from build123d import *

# Parameters (mm, degrees)
SKETCH1_W               = 50
SKETCH1_H               = 50
BODY_DEPTH              = 10
SKETCH2_R               = 11.5
CUT_VIEW_DEPTH          = 7
FILLETBODY_R            = 3
SKETCH3_R               = 3.75
BOLT_EXTRUDE_DEPTH      = 1
SKETCH4_R               = 1.5
BOLT_DEPTH              = 10
BOLT_DEPTH_BACK         = 16
HEX_2_DEPTH             = 2
SKETCH19_R              = 1.5
HEX_BOLT_DEPTH          = 3
SKETCH6_R               = 4
FIELD1_DEPTH            = 7
FIELD2_R                = 4
SKETCH7_R               = 2.575
PORTS1_DEPTH            = 12
SKETCH10_R              = 1.575
PORTS2_DEPTH            = 12
PORTS2_DEPTH_BACK       = 32
SKETCH11_R              = 20
SKETCH11_R_2            = 15
SEAL1_DEPTH             = 0.5
FLOWFIELD_DEPTH         = 1.5
FLOWFIELD_CHANNEL_DEPTH = 1.5
BODY_MOVE_COPY1_ANGLE   = 90
BODY_MOVE_COPY2_ANGLE   = 180
SKETCH20_R              = 2.575
CUT_EXTRUDE1_DEPTH      = 17
FILLET1_R               = 0.5


with BuildPart() as part:
    # Sketch1 → Body (new body)
    with BuildSketch(Plane(origin=(0, 0, 0), x_dir=(1, 0, 0), z_dir=(0, 1, 0))):
        Rectangle(SKETCH1_W, SKETCH1_H)
    extrude(amount=BODY_DEPTH)

    # Sketch2 → Cut view (cut)
    with BuildSketch(Plane(origin=(0, 10, 0), x_dir=(1, 0, 0), z_dir=(0, 1, 0))):
        Circle(SKETCH2_R)
    extrude(amount=-CUT_VIEW_DEPTH, mode=Mode.SUBTRACT)

    # FilletBody
    filletbody_edges = [part.edges().sort_by_distance(p)[0] for p in [
        (-25, 5, -25),
        (25, 5, -25),
        (25, 5, 25),
        (-25, 5, 25),
    ]]
    fillet(filletbody_edges, radius=FILLETBODY_R)

    # Sketch3 → Bolt extrude (add)
    with BuildSketch(Plane(origin=(0, 10, 0), x_dir=(1, 0, 0), z_dir=(0, 1, 0))):
        with Locations((-17.5, 17.5)):
            Circle(SKETCH3_R)
        with Locations((17.5, 17.5)):
            Circle(SKETCH3_R)
        with Locations((17.5, -17.5)):
            Circle(SKETCH3_R)
        with Locations((-17.5, -17.5)):
            Circle(SKETCH3_R)
    extrude(amount=BOLT_EXTRUDE_DEPTH)

    # Sketch4 → Bolt (cut, two sides)
    with BuildSketch(Plane(origin=(0, 11, 0), x_dir=(1, 0, 0), z_dir=(0, 1, 0))) as bolt_sk:
        with Locations((-17.5, 17.5)):
            Circle(SKETCH4_R)
        with Locations((17.5, 17.5)):
            Circle(SKETCH4_R)
        with Locations((17.5, -17.5)):
            Circle(SKETCH4_R)
        with Locations((-17.5, -17.5)):
            Circle(SKETCH4_R)
    extrude(amount=BOLT_DEPTH, mode=Mode.SUBTRACT)
    extrude(bolt_sk.sketch, amount=-BOLT_DEPTH_BACK, mode=Mode.SUBTRACT)

    # Sketch5 → Hex 2 (cut)
    with BuildSketch(Plane(origin=(0, 10, 0), x_dir=(1, 0, 0), z_dir=(0, 1, 0))):
        Polygon((0, 22.233161507), (-2.8, 20.616580754), (-2.8, 17.383419246), (0, 15.766838493), (2.8, 17.383419246), (2.8, 20.616580754), align=None)
    extrude(amount=-HEX_2_DEPTH, mode=Mode.SUBTRACT)

    # Sketch19 → Hex_bolt (cut)
    with BuildSketch(Plane(origin=(0, 8, 0), x_dir=(1, 0, 0), z_dir=(0, 1, 0))):
        with Locations((0, 19)):
            Circle(SKETCH19_R)
    extrude(amount=-HEX_BOLT_DEPTH, mode=Mode.SUBTRACT)

    # Sketch6 → Field1 (add)
    with BuildSketch(Plane(origin=(0, 10, 0), x_dir=(1, 0, 0), z_dir=(0, 1, 0))):
        with Locations((-13, 0)):
            Circle(SKETCH6_R)
        with Locations((13, 0)):
            Circle(SKETCH6_R)
    extrude(amount=-FIELD1_DEPTH)

    # Field2
    field2_edges = [part.edges().sort_by_distance(p)[0] for p in [
        (-10.971153846, 6.5, 3.447286365),
        (-10.971153846, 6.5, -3.447286365),
        (10.971153846, 6.5, -3.447286365),
        (10.971153846, 6.5, 3.447286365),
    ]]
    fillet(field2_edges, radius=FIELD2_R)

    # Sketch7 → Ports1 (add)
    with BuildSketch(Plane(origin=(0, 10, 0), x_dir=(1, 0, 0), z_dir=(0, 1, 0))):
        with Locations((-13, 0)):
            Circle(SKETCH7_R)
        with Locations((13, 0)):
            Circle(SKETCH7_R)
    extrude(amount=PORTS1_DEPTH)

    # Sketch10 → Ports2 (cut, two sides)
    with BuildSketch(Plane(origin=(0, 22, 0), x_dir=(1, 0, 0), z_dir=(0, 1, 0))) as ports2_sk:
        with Locations((-13, 0)):
            Circle(SKETCH10_R)
        with Locations((13, 0)):
            Circle(SKETCH10_R)
    extrude(amount=PORTS2_DEPTH, mode=Mode.SUBTRACT)
    extrude(ports2_sk.sketch, amount=-PORTS2_DEPTH_BACK, mode=Mode.SUBTRACT)

    # Sketch11 → Seal1 (cut)
    with BuildSketch(Plane.XZ):
        Circle(SKETCH11_R)
        Circle(SKETCH11_R_2, mode=Mode.SUBTRACT)
    extrude(amount=-SEAL1_DEPTH, mode=Mode.SUBTRACT)

    # Sketch15 → FlowField (cut)
    with BuildSketch(Plane.XZ):
        with BuildLine():
            ThreePointArc((13.522961568, 3.623466631), (-1.199537572, 13.948516395), (-13.943052885, 1.261457989))
            ThreePointArc((-13.943052885, 1.261457989), (-12.926234652, 1.573271646), (-11.943052885, 1.167684801))
            ThreePointArc((-11.943052885, 1.167684801), (-0.984919414, 11.95951227), (11.591109915, 3.105828541))
            ThreePointArc((11.591109915, 3.105828541), (12.815854787, 2.39872176), (13.522961568, 3.623466631))
        make_face()
        with BuildLine():
            ThreePointArc((11, 0), (1.910129954, 10.832885283), (-10.336618829, 3.762221577))
            ThreePointArc((-10.336618829, 3.762221577), (-9.738946351, 2.480508812), (-8.457233587, 3.07818129))
            ThreePointArc((-8.457233587, 3.07818129), (1.562833599, 8.863269777), (9, 0))
            Line((9, 0), (11, 0))
        make_face()
        with BuildLine():
            ThreePointArc((7.250462296, 3.380946094), (6.766772771, 2.052020045), (5.437846722, 2.53570957))
            ThreePointArc((5.437846722, 2.53570957), (-1.298637684, 5.857776043), (-6, 0))
            Line((-6, 0), (-8, 0))
            ThreePointArc((-8, 0), (-1.731516912, 7.810368057), (7.250462296, 3.380946094))
        make_face()
        with BuildLine():
            ThreePointArc((5, 0), (1.913417162, 4.619397663), (-3.535533906, 3.535533906))
            ThreePointArc((-3.535533906, 3.535533906), (-3.535533906, 2.121320344), (-2.121320344, 2.121320344))
            ThreePointArc((-2.121320344, 2.121320344), (1.148050297, 2.771638598), (3, 0))
            Line((3, 0), (5, 0))
        make_face()
        with BuildLine():
            ThreePointArc((5, 0), (1.913417162, -4.619397663), (-3.535533906, -3.535533906))
            ThreePointArc((-3.535533906, -3.535533906), (-3.535533906, -2.121320344), (-2.121320344, -2.121320344))
            ThreePointArc((-2.121320344, -2.121320344), (1.148050297, -2.771638598), (3, 0))
            Line((3, 0), (5, 0))
        make_face()
        with BuildLine():
            ThreePointArc((-8, 0), (-1.731516912, -7.810368057), (7.250462296, -3.380946094))
            ThreePointArc((7.250462296, -3.380946094), (6.766772771, -2.052020045), (5.437846722, -2.53570957))
            ThreePointArc((5.437846722, -2.53570957), (-1.298637684, -5.857776043), (-6, 0))
            Line((-6, 0), (-8, 0))
        make_face()
        with BuildLine():
            ThreePointArc((11, 0), (1.910129954, -10.832885283), (-10.336618829, -3.762221577))
            ThreePointArc((-10.336618829, -3.762221577), (-9.738946351, -2.480508812), (-8.457233587, -3.07818129))
            ThreePointArc((-8.457233587, -3.07818129), (1.562833599, -8.863269777), (9, 0))
            Line((9, 0), (11, 0))
        make_face()
        with BuildLine():
            ThreePointArc((-11.943052885, -1.167684801), (-12.926234652, -1.573271646), (-13.943052885, -1.261457989))
            ThreePointArc((-13.943052885, -1.261457989), (-1.199537572, -13.948516395), (13.522961568, -3.623466631))
            ThreePointArc((13.522961568, -3.623466631), (12.815854787, -2.39872176), (11.591109915, -3.105828541))
            ThreePointArc((11.591109915, -3.105828541), (-0.984919414, -11.95951227), (-11.943052885, -1.167684801))
        make_face()
    extrude(amount=-FLOWFIELD_DEPTH, mode=Mode.SUBTRACT)

    # Sketch16 → FlowField_Channel (cut)
    with BuildSketch(Plane.XZ):
        with BuildLine():
            Line((-13, 1), (0, 1))
            ThreePointArc((0, 1), (1, 0), (0, -1))
            Line((0, -1), (-13, -1))
            ThreePointArc((-13, -1), (-14, 0), (-13, 1))
        make_face()
        with BuildLine():
            Line((13, -1), (4.429119544, -1))
            ThreePointArc((4.429119544, -1), (3.429119544, 0), (4.429119544, 1))
            Line((4.429119544, 1), (13, 1))
            ThreePointArc((13, 1), (14, 0), (13, -1))
        make_face()
    extrude(amount=-FLOWFIELD_CHANNEL_DEPTH, mode=Mode.SUBTRACT)


with BuildPart() as body_2:
    # Mirror3: mirrored copy
    add(part.part.mirror(Plane.ZX))


with BuildPart() as body_2_1:
    # Body-Move/Copy1: moved
    add(body_2.part.rotate(Axis((0, -11, 0), (-1, 0, 0)), BODY_MOVE_COPY1_ANGLE))


with BuildPart() as body_2_2:
    # Body-Move/Copy2: moved
    add(body_2_1.part.rotate(Axis((0, -11, 0), (0, 0, 1)), BODY_MOVE_COPY2_ANGLE))

    # Sketch20 → Cut-Extrude1 (cut)
    with BuildSketch(Plane.XY.offset(11)):
        with Locations((-13, -11)):
            Circle(SKETCH20_R)
        with Locations((13, -11)):
            Circle(SKETCH20_R)
    extrude(amount=-CUT_EXTRUDE1_DEPTH, mode=Mode.SUBTRACT)

    # Fillet1
    fillet1_edges = [body_2_2.edges().sort_by_distance(p)[0] for p in [
        (0, 11.233161507, -2),
        (-2.8, 9.616580754, -2),
        (-2.8, 6.383419246, -2),
        (0, 4.766838493, -2),
        (2.8, 6.383419246, -2),
        (2.8, 9.616580754, -2),
    ]]
    fillet(fillet1_edges, radius=FILLET1_R)


solid = body_2_2.part
Input: part model. Units: mm. Frame: model coordinates. A direction names the side the tool comes from. Give positions to 0.01 mm unless a question says otherwise; leave off trailing zeros. Write each loop counter-clockwise with the first axis right and the second up, starting at its lowest first coordinate (ties: lowest second). Pieces come first, ordered by that corner, then holes. Notation, with made-up numbers: M -12.75,22 L 42.25,22 A29 ccw 42.25,54 Z; hole C 47,3 d3. An arc over 180 degrees is marked long. Use one line per item in the form item = value.
1. Cut plane A-A on x = 13. Return loops of the section in (y, z) (3 decimals).
Outcome:
outline = M -36,-11 L -26.199,-11 L -26.199,-10.5 L -18.483,-10.5 L -18.483,-11 L -16.196,-11 L -16.196,-9.5 L -12.575,-9.5 L -12.575,-6 L -13.575,-6 L -13.575,-1 L -36,-1 Z; M -9.425,-9.5 L -5.804,-9.5 L -5.804,-11 L -3.517,-11 L -3.517,-10.5 L 4.199,-10.5 L 4.199,-11 L 14,-11 L 14,-1 L -8.425,-1 L -8.425,-6 L -9.425,-6 Z
2. Ray query, L1, parallel to Y at x = 17.5, z = -6; L2, parallel to Y at x = 0, z = -3.9; L3, parallel to X at y = -11, z = -4.3 (3 decimals). Return the intervals inside material, ascending.
Outcome:
L1 = -36 to -30, -27 to 5, 8 to 14
L2 = -36 to -22.5, 0.5 to 6.5, 9.5 to 14
L3 = -25 to -15.575, -10.425 to -9, 9 to 10.425, 15.575 to 25
3. Reachability of faces 1 (the face through (-1.416, 10.416, -1.986)), 2 (the face through (-12.795, -13.393, -10.26)), 3 (the face through (0, -9, -11)) from +Z, -Z, +X, -X, +Y, -Y: full face, straight path, thin tool, end or side. Return the list, or none.
Outcome:
face_1 = +Z
face_2 = -Z
face_3 = -Z, +X, -X, +Y, -Y
4. Mould query, pull axis X, two halves, no side actions, for faces 4 (the face through (-7, -10, -10)), 5 (the face through (16.7, 4.9, 0)). Classes: released by +X, released by -X, zero draft, split by the parting line, or undercut.
Outcome:
face_4 = undercut
face_5 = zero draft
5. First-contact query: P1, Ø8, axis at x = 13, y = -11, coming from the +Z side; P2, Ø0.9, axis at x = 0, y = 8.5, coming from the +Z side; P3, Ø4, axis at x = 11.5, y = -24.5, coming from the -Z side. Flat tips, straight axial feed; report the tip coordinate or a pass-through.
Outcome:
P1 = -1
P2 = -6
P3 = -10.5
